Here's the drawing with two shaded views (mm, measured from the low corner). I have some questions. A direction names the side the tool comes from. Coordinates: 2 decimals unless noted, no trailing zeros. Loops run counter-clockwise (first coordinate to the right, second up) from the corner with the lowest first, then second, coordinate; pieces in that order, holes last. Notation, with made-up numbers: (-9, -9.75) -> (32, -9.75) arc R9 ccw to (32, -2.75) -> close; hole circle Ø3 at (64.5, 61.5). An arc over 180 degrees is marked (long way). Answer as a JSON object with one key per item and string values. Group by question number.
Q1. I need wall thicknesses on line 1 (Y direction, x = 88, z = 33.5); line 2 (Z direction, x = 84.5, y = 32); line 3 (X direction, y = 12, z = 29). Which ranges of each line are inside material? Lowest first, please.
Q2. I want a section at C-C on x = 93. Write out the boundary of the cut face in (y, z), then the cut area to 3 significant figures.
Q3. I want a section at D-D on y = 9. Write out the boundary of the cut face in (x, z).
Q4. I want a section at A-A on y = 31. Write out the boundary of the cut face in (x, z).
Q5. I want a section at B-B on z = 40.5. Write out the boundary of the cut face in (x, y), then the cut area to 3 significant figures.
Q6. On a 3-axis mill with a long thin cutter (end or side, diameter ignored), from which of +Z, -Z, +X, -X, +Y, -Y can I reach the whole of each face in a straight line? I mean the marked faces 1 and 2. Say none if no direction works.
Q7. I'm going to push flat-ended pins straight in: pin 1 (2 mm diameter, centred on x = 84, y = 20.5, fed in from +Z); pin 2 (10 mm diameter, centred on y = 31.5, z = 35.5, fed in from -X); pin 3 (12 mm diameter, centred on x = 55, y = 27, fed in from -Z); pin 4 (1 mm diameter, centred on x = 83, z = 13, fed in from +Y). Where does each tip first touch, or does it pass through?
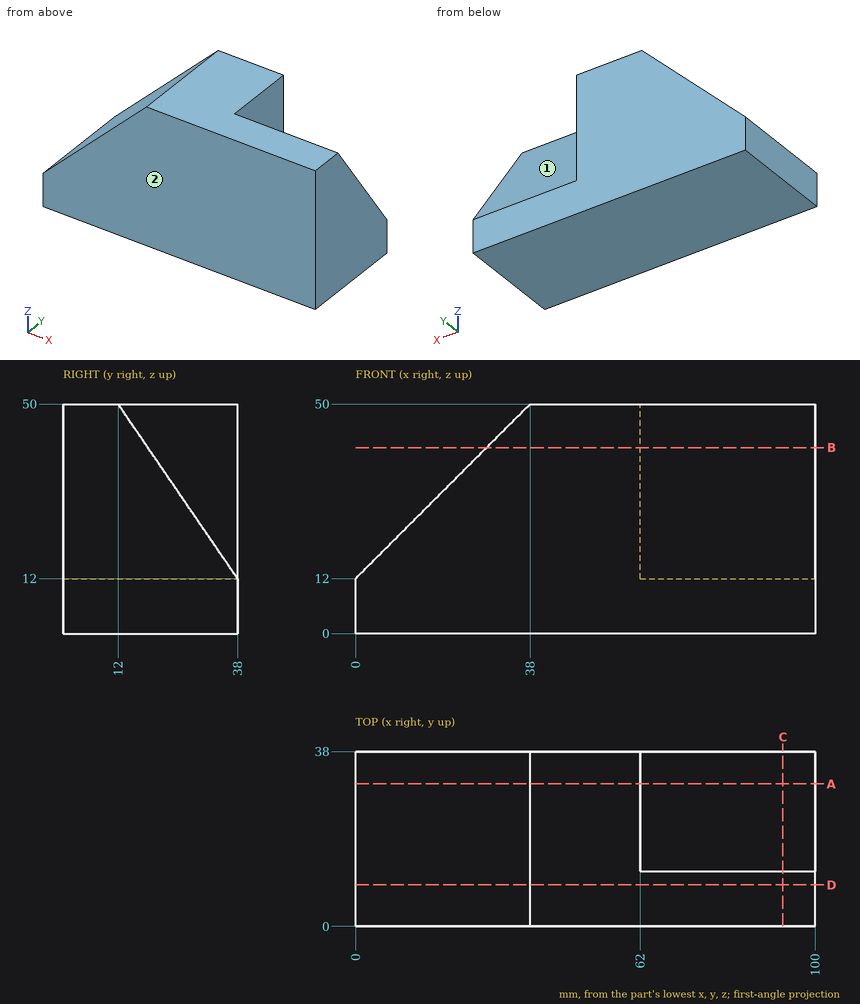
Result set:
{
 "1": {"line 1": "y = 0 to 23.29", "line 2": "z = 0 to 20.77", "line 3": "x = 17 to 100"},
 "2": {"outline": "(0, 0) -> (38, 0) -> (38, 12) -> (12, 50) -> (0, 50) -> close", "area": "1,410 mm²"},
 "3": {"outline": "(0, 0) -> (100, 0) -> (100, 50) -> (38, 50) -> (0, 12) -> close"},
 "4": {"outline": "(0, 0) -> (100, 0) -> (100, 22.23) -> (62, 22.23) -> (62, 50) -> (38, 50) -> (0, 12) -> close"},
 "5": {"outline": "(28.5, 0) -> (100, 0) -> (100, 18.5) -> (62, 18.5) -> (62, 38) -> (28.5, 38) -> close", "area": "1,980 mm²"},
 "6": {"face 1": "+Z, +X, +Y", "face 2": "+Z, -Z, +X, -X, -Y"},
 "7": {"pin 1": "stops at z = 39.04", "pin 2": "stops at x = 18.5", "pin 3": "stops at z = 0", "pin 4": "stops at y = 37.66"}
}
